Check sheet for the modelled part. Datum: model origin and axes. Units: mm. A direction names the side the tool comes from. Coordinates: 2 decimals unless noted, no trailing zeros. Write each loop counter-clockwise with the first axis right and the second up, starting at its lowest first coordinate (ties: lowest second). Pieces come first, ordered by that corner, then holes. Notation, with made-up numbers: (9.5, -1.5) -> (28.5, -1.5) arc R33 cw to (28.5, 27.5) -> close; hole circle Ø6 at (44, -16). An arc over 180 degrees is marked (long way). One line per item, written item: value. Start each with the question number.
1) Sectioned sample at B-B on z = 4. Enter the section's corners in (x, y) (3 decimals).
2) Scan lines: line 1 along Y through (x, z) = (3, 8.75); line 2 along Z through (x, y) = (2.75, -12.25). Record each from-to range of solid material in increasing order. Write a range as [from, to].
3) Draft check along Y on faces 1 (the flat face through (5, 0, 8)), 2 (the cylindrical face through (4.83, 0.45, 17.07)), 3 (the cylindrical face through (5.01, -10, 17.04)). Enter one of: +Y half, -Y half, draft (parallel to the pull), parting line (faces both ways), or undercut.
4) Sectioned sample at D-D on x = 8. Enter the section's corners in (y, z), plus the area to 3 significant figures.
5) Sectioned sample at C-C on x = 3.5. Enter the section's corners in (y, z).
6) Set-up check for faces 4 (the cylindrical face through (0.362, -16.255, 17.038)), 5 (the flat face through (5, -8, 16.637)): record each of +Z, -Z, +X, -X, +Y, -Y from which the full face is reachable in a straight line by a thin tool's end or side.
7) Gauge pin test, flat ends, axial feed: P1, Ø3, axis at x = 3, y = -10.5, coming from the -Z side; P2, Ø3, axis at x = 7.5, z = 14, coming from the -Y side. Record the tip position at first contact, or that the pin passes through.
8) Sectioned sample at A-A on y = -13.25. Enter the section's corners in (x, z) (3 decimals), plus the area to 3 significant figures.
```python
from build123d import *

# Parameters (mm, degrees)
SKETCH1_W           = 9.525
SKETCH1_H           = 0.8128
BOSS_EXTRUDE1_DEPTH = 17.4498
SKETCH2_W           = 9.525
SKETCH2_H           = 0.8128
BOSS_EXTRUDE2_DEPTH = 17.4498
SKETCH3_R           = 1.905
CUT_EXTRUDE1_DEPTH  = 17.4498
SKETCH4_R           = 1.905
CUT_EXTRUDE2_DEPTH  = 17.4498
FILLET1_R           = 1.27


with BuildPart() as part:
    # Sketch1 → Boss-Extrude1 (new body)
    with BuildSketch(Plane.XY):
        with Locations((4.7625, 0.4064)):
            Rectangle(SKETCH1_W, SKETCH1_H)
    extrude(amount=BOSS_EXTRUDE1_DEPTH)

    # Sketch2 → Boss-Extrude2 (add)
    with BuildSketch(Plane(origin=(0, 0.8128, 0), x_dir=(1, 0, 0), z_dir=(0, 1, 0))):
        with Locations((4.7625, -17.0434)):
            Rectangle(SKETCH2_W, SKETCH2_H)
    extrude(amount=-BOSS_EXTRUDE2_DEPTH)

    # Sketch3 → Cut-Extrude1 (cut)
    with BuildSketch(Plane.XZ):
        with Locations(Location((4.7625, 4.7498, 0), (0, 0, 270))):
            Circle(SKETCH3_R)
    extrude(amount=-CUT_EXTRUDE1_DEPTH, mode=Mode.SUBTRACT)

    # Sketch4 → Cut-Extrude2 (cut)
    with BuildSketch(Plane(origin=(0, 0, 16.637), x_dir=(-1, 0, 0), z_dir=(0, 0, -1))):
        with Locations((-4.7625, -11.8872)):
            Circle(SKETCH4_R)
    extrude(amount=-CUT_EXTRUDE2_DEPTH, mode=Mode.SUBTRACT)

    # Fillet1
    fillet1_edges = [part.edges().sort_by_distance(p)[0] for p in [
        (4.7625, 0.8128, 17.4498),
        (0, -16.637, 17.0434),
        (9.525, -16.637, 17.0434),
        (9.525, 0.4064, 0),
        (0, 0.4064, 0),
    ]]
    fillet(fillet1_edges, radius=FILLET1_R)


solid = part.part
```
Answers:
1. outline: (0, 0) -> (3.011, 0) -> (3.011, 0.813) -> (0, 0.813) -> close; (6.514, 0) -> (9.525, 0) -> (9.525, 0.813) -> (6.514, 0.813) -> close
2. line 1: y = [0, 0.81]
2. line 2: z = [16.64, 17.45]
3. face 1: -Y half
3. face 2: +Y half
3. face 3: undercut
4. outline: (-16.64, 16.64) -> (0, 16.64) -> (0, 0) -> (0.81, 0) -> (0.81, 16.18) arc R1.27 ccw to (-0.46, 17.45) -> (-16.64, 17.45) -> close
4. area: 27.4 mm2
5. outline: (-16.64, 16.64) -> (-13.31, 16.64) -> (-13.31, 17.45) -> (-16.64, 17.45) -> close; (-10.46, 16.64) -> (0, 16.64) -> (0, 6.18) -> (0.81, 6.18) -> (0.81, 16.18) arc R1.27 ccw to (-0.46, 17.45) -> (-10.46, 17.45) -> close; (0, 0) -> (0.81, 0) -> (0.81, 3.32) -> (0, 3.32) -> close
6. face 4: +Z, -Z, -X, -Y
6. face 5: -Z, +X, -X, -Y
7. P1: stops at z = 16.64
7. P2: stops at y = 0
8. outline: (0, 16.637) -> (3.431, 16.637) -> (3.431, 17.45) -> (0, 17.45) -> close; (6.094, 16.637) -> (9.525, 16.637) -> (9.525, 17.45) -> (6.094, 17.45) -> close
8. area: 5.58 mm2
